from build123d import *

# Parameters (mm, degrees)
SKETCH1_W           = 50.8
SKETCH1_H           = 57.15
SKETCH1_W_2         = 2.54
SKETCH1_H_2         = 55.88
SKETCH1_W_3         = 10.16
BOSS_EXTRUDE1_DEPTH = 3.175
BOSS_EXTRUDE2_DEPTH = 6.35
SKETCH3_R           = 1.651
CUT_EXTRUDE1_DEPTH  = 49.568160867
CUT_EXTRUDE2_DEPTH  = 49.568160867


with BuildPart() as part:
    # Sketch1 → Boss-Extrude1 (new body)
    with BuildSketch(Plane(origin=(0, 0, 0), x_dir=(1, 0, 0), z_dir=(0, 1, 0))):
        Rectangle(SKETCH1_W, SKETCH1_H)
        with Locations((-26.67, 0)):
            Rectangle(SKETCH1_W_2, SKETCH1_H_2)
        with Locations((-33.02, 0)):
            Rectangle(SKETCH1_W_3, SKETCH1_H_2)
    extrude(amount=BOSS_EXTRUDE1_DEPTH)

    # Sketch2 → Boss-Extrude2 (add)
    with BuildSketch(Plane.XZ):
        Polygon((-27.94, 6.892407514), (-28.702, 7.332348419), (-35.052, 3.666174209), (-35.052, -3.666174209), (-28.702, -7.332348419), (-27.94, -6.892407514), align=None)
        Polygon((-35.052, 27.94), (-35.052, 21.733825791), (-28.702, 18.067651581), (-27.94, 18.507592486), (-27.94, 27.94), align=None)
        Polygon((-27.94, -18.507592486), (-27.94, -27.94), (-35.052, -27.94), (-35.052, -21.733825791), (-28.702, -18.067651581), align=None)
    extrude(amount=BOSS_EXTRUDE2_DEPTH)

    # Sketch3 → Cut-Extrude1 (cut, through all)
    with BuildSketch(Plane(origin=(0, 3.175, 0), x_dir=(1, 0, 0), z_dir=(0, 1, 0))):
        with Locations(Location((20.7772, -24.003, 0), (0, 0, 270))):
            Circle(SKETCH3_R)
        with Locations(Location((14.4272, -24.003, 0), (0, 0, 270))):
            Circle(SKETCH3_R)
        with Locations(Location((8.0772, -24.003, 0), (0, 0, 270))):
            Circle(SKETCH3_R)
        with Locations(Location((1.7272, -24.003, 0), (0, 0, 270))):
            Circle(SKETCH3_R)
        with Locations(Location((-4.6228, -24.003, 0), (0, 0, 270))):
            Circle(SKETCH3_R)
        with Locations(Location((-10.9728, -24.003, 0), (0, 0, 270))):
            Circle(SKETCH3_R)
        with Locations(Location((-17.3228, -24.003, 0), (0, 0, 270))):
            Circle(SKETCH3_R)
        with Locations(Location((-23.6728, -24.003, 0), (0, 0, 270))):
            Circle(SKETCH3_R)
        with Locations(Location((-23.6728, 24.003, 0), (0, 0, 270))):
            Circle(SKETCH3_R)
        with Locations(Location((-17.3228, 24.003, 0), (0, 0, 270))):
            Circle(SKETCH3_R)
        with Locations(Location((-10.9728, 24.003, 0), (0, 0, 270))):
            Circle(SKETCH3_R)
        with Locations(Location((-4.6228, 24.003, 0), (0, 0, 270))):
            Circle(SKETCH3_R)
        with Locations(Location((1.7272, 24.003, 0), (0, 0, 270))):
            Circle(SKETCH3_R)
        with Locations(Location((8.0772, 24.003, 0), (0, 0, 270))):
            Circle(SKETCH3_R)
        with Locations(Location((14.4272, 24.003, 0), (0, 0, 270))):
            Circle(SKETCH3_R)
        with Locations(Location((20.7772, 24.003, 0), (0, 0, 270))):
            Circle(SKETCH3_R)
    extrude(amount=-CUT_EXTRUDE1_DEPTH, mode=Mode.SUBTRACT)

    # Sketch4 → Cut-Extrude2 (cut, through all)
    with BuildSketch(Plane(origin=(0, 3.175, 0), x_dir=(1, 0, 0), z_dir=(0, 1, 0))):
        Polygon((17.634991976, 18.279152345), (22.579981612, 18.279152345), (22.579981612, 21.200152345), (15.94855184, 21.200152345), align=None)
        Polygon((16.232450896, 17.517152345), (14.106069855, 21.200152345), (6.627074468, 21.200152345), (4.500693426, 17.517152345), (7.433632794, 12.437152345), (13.299511529, 12.437152345), align=None)
        Polygon((3.180870711, 18.279152345), (4.867310847, 21.200152345), (-4.37144816, 21.200152345), (-2.685008024, 18.279152345), align=None)
        Polygon((-4.087549104, 17.517152345), (-6.213930145, 21.200152345), (-13.692925532, 21.200152345), (-15.819306574, 17.517152345), (-12.886367206, 12.437152345), (-7.020488471, 12.437152345), align=None)
        Polygon((-17.139129289, 18.279152345), (-15.452689153, 21.200152345), (-24.641954227, 21.200152345), (-24.641954227, 21.114426338), (-23.005008024, 18.279152345), align=None)
        Polygon((-23.005008024, 16.755152345), (-24.641954227, 13.919878353), (-24.641954227, 9.430426338), (-23.005008024, 6.595152345), (-17.139129289, 6.595152345), (-14.206189922, 11.675152345), (-17.139129289, 16.755152345), align=None)
        Polygon((-23.005008024, 5.071152345), (-24.641954227, 2.235878353), (-24.641954227, -2.253573662), (-23.005008024, -5.088847655), (-17.139129289, -5.088847655), (-14.206189922, -0.008847655), (-17.139129289, 5.071152345), align=None)
        Polygon((-24.641954227, -9.448121647), (-24.641954227, -13.937573662), (-23.005008024, -16.772847655), (-17.139129289, -16.772847655), (-14.206189922, -11.692847655), (-17.139129289, -6.612847655), (-23.005008024, -6.612847655), align=None)
        Polygon((-24.641954227, -21.217847655), (-15.452689153, -21.217847655), (-17.139129289, -18.296847655), (-23.005008024, -18.296847655), (-24.641954227, -21.132121647), align=None)
        Polygon((-13.692925532, -21.217847655), (-6.213930145, -21.217847655), (-4.087549104, -17.534847655), (-7.020488471, -12.454847655), (-12.886367206, -12.454847655), (-15.819306574, -17.534847655), align=None)
        Polygon((-4.37144816, -21.217847655), (4.867310847, -21.217847655), (3.180870711, -18.296847655), (-2.685008024, -18.296847655), align=None)
        Polygon((6.627074468, -21.217847655), (14.106069855, -21.217847655), (16.232450896, -17.534847655), (13.299511529, -12.454847655), (7.433632794, -12.454847655), (4.500693426, -17.534847655), align=None)
        Polygon((22.579981612, -21.217847655), (22.579981612, -18.296847655), (17.634991976, -18.296847655), (15.94855184, -21.217847655), align=None)
        Polygon((22.579981612, -16.772847655), (22.579981612, -6.612847655), (17.634991976, -6.612847655), (14.702052608, -11.692847655), (17.634991976, -16.772847655), align=None)
        Polygon((22.579981612, -5.088847655), (22.579981612, 5.071152345), (17.634991976, 5.071152345), (14.702052608, -0.008847655), (17.634991976, -5.088847655), align=None)
        Polygon((17.634991976, 6.595152345), (22.579981612, 6.595152345), (22.579981612, 16.755152345), (17.634991976, 16.755152345), (14.702052608, 11.675152345), align=None)
        Polygon((4.500693426, 5.833152345), (7.433632794, 0.753152345), (13.299511529, 0.753152345), (16.232450896, 5.833152345), (13.299511529, 10.913152345), (7.433632794, 10.913152345), align=None)
        Polygon((-2.685008024, 6.595152345), (3.180870711, 6.595152345), (6.113810078, 11.675152345), (3.180870711, 16.755152345), (-2.685008024, 16.755152345), (-5.617947392, 11.675152345), align=None)
        Polygon((-2.685008024, -5.088847655), (3.180870711, -5.088847655), (6.113810078, -0.008847655), (3.180870711, 5.071152345), (-2.685008024, 5.071152345), (-5.617947392, -0.008847655), align=None)
        Polygon((4.500693426, -5.850847655), (7.433632794, -10.930847655), (13.299511529, -10.930847655), (16.232450896, -5.850847655), (13.299511529, -0.770847655), (7.433632794, -0.770847655), align=None)
        Polygon((-2.685008024, -16.772847655), (3.180870711, -16.772847655), (6.113810078, -11.692847655), (3.180870711, -6.612847655), (-2.685008024, -6.612847655), (-5.617947392, -11.692847655), align=None)
        Polygon((-15.819306574, -5.850847655), (-12.886367206, -10.930847655), (-7.020488471, -10.930847655), (-4.087549104, -5.850847655), (-7.020488471, -0.770847655), (-12.886367206, -0.770847655), align=None)
        Polygon((-15.819306574, 5.833152345), (-12.886367206, 0.753152345), (-7.020488471, 0.753152345), (-4.087549104, 5.833152345), (-7.020488471, 10.913152345), (-12.886367206, 10.913152345), align=None)
    extrude(amount=-CUT_EXTRUDE2_DEPTH, mode=Mode.SUBTRACT)


solid = part.part
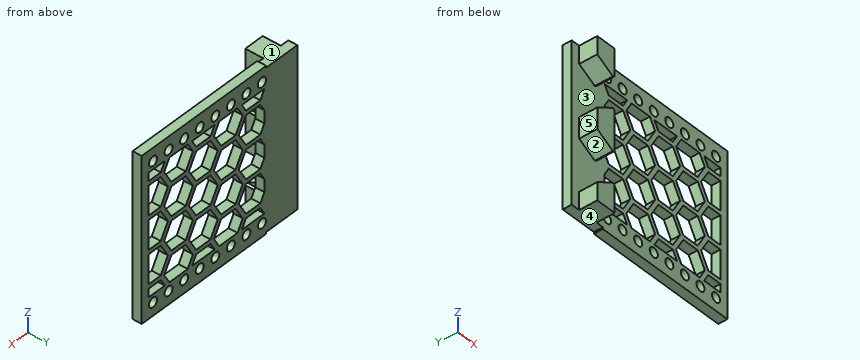
Design review of the part built by this model. Coordinates are the model's own, in mm. Face numbers are marked on the shaded views. A direction names the side the tool comes from. Coordinates: 2 decimals unless noted, no trailing zeros. Loops run counter-clockwise (first coordinate to the right, second up) from the corner with the lowest first, then second, coordinate; pieces in that order, holes last. Notation, with made-up numbers: (49, -16.75) -> (100, -16.75) arc R24 cw to (100, 12.25) -> close; hole circle Ø1 at (-6.75, -7.75). An arc over 180 degrees is marked (long way). Use a Markdown table: item, result. Add a question column.
Item 1: Wall thickness on L1, parallel to X at y = 1, z = 4; L2, parallel to X at y = 2, z = 5.5; L3, parallel to X at y = 0.5, z = 17: over which ranges is each line inside the solid? List them lowest first. Write a range as from..to.
Item 2: We need section B-B, the plane y = 2. Count the separate pieces of the cut face and the enclosed holes in it, and give its area (3 significant figures).
Item 3: Clearance check with flat-ended pins moving along their axes: P1, Ø2, axis at x = 20.78, z = -24, coming from the -Y side; P2, Ø4, axis at x = -4.62, z = -24, coming from the -Y side; P3, Ø2, axis at y = -3.5, z = 17.5, coming from the -X side; P4, Ø0.5, axis at y = 1.5, z = -28.5, coming from the -X side. State where each tip first meets the part, or that it passes through.
Item 4: Machinability: for the marked faces 1, 2, 3, 4 and 5, which of the approach directions +Z, -Z, +X, -X, +Y, -Y give a long, thin tool a straight path to every point of the face, cutting with its end or side? Answer none if there is none.
Item 5: We need section A-A, the plane y = -1.75. Write out the cut boundary in (x, z).
Numbers:
| question | item | result |
|---|---|---|
| 1 | L1 | x = -38.1..-23.63, -16.51..-14.75, -5.16..-3.31, 3.81..5.57, 15.16..17.01, 22.58..25.4 |
| 1 | L2 | x = -38.1..-15.62, -4.29..4.7, 16.03..25.4 |
| 1 | L3 | x = -38.1..-15.51, -4.4..4.81, 15.92..25.4 |
| 2 | separate pieces | 1 |
| 2 | enclosed holes | 39 |
| 2 | area | 1,950 mm^2 |
| 3 | P1 | passes through |
| 3 | P2 | stops at y = 0 |
| 3 | P3 | stops at x = -29.45 |
| 3 | P4 | stops at x = -25.4 |
| 4 | face 1 | +Z, -X, +Y, -Y |
| 4 | face 2 | -X, -Y |
| 4 | face 3 | -Y |
| 4 | face 4 | -Z, -X, +Y, -Y |
| 4 | face 5 | +Z, -Z, -X, -Y |
| 5 | outline | (-35.05, -27.94) -> (-27.94, -27.94) -> (-27.94, -18.51) -> (-28.7, -18.07) -> (-35.05, -21.73) -> close; (-35.05, -3.67) -> (-28.7, -7.33) -> (-27.94, -6.89) -> (-27.94, 6.89) -> (-28.7, 7.33) -> (-35.05, 3.67) -> close; (-35.05, 21.73) -> (-28.7, 18.07) -> (-27.94, 18.51) -> (-27.94, 27.94) -> (-35.05, 27.94) -> close |
